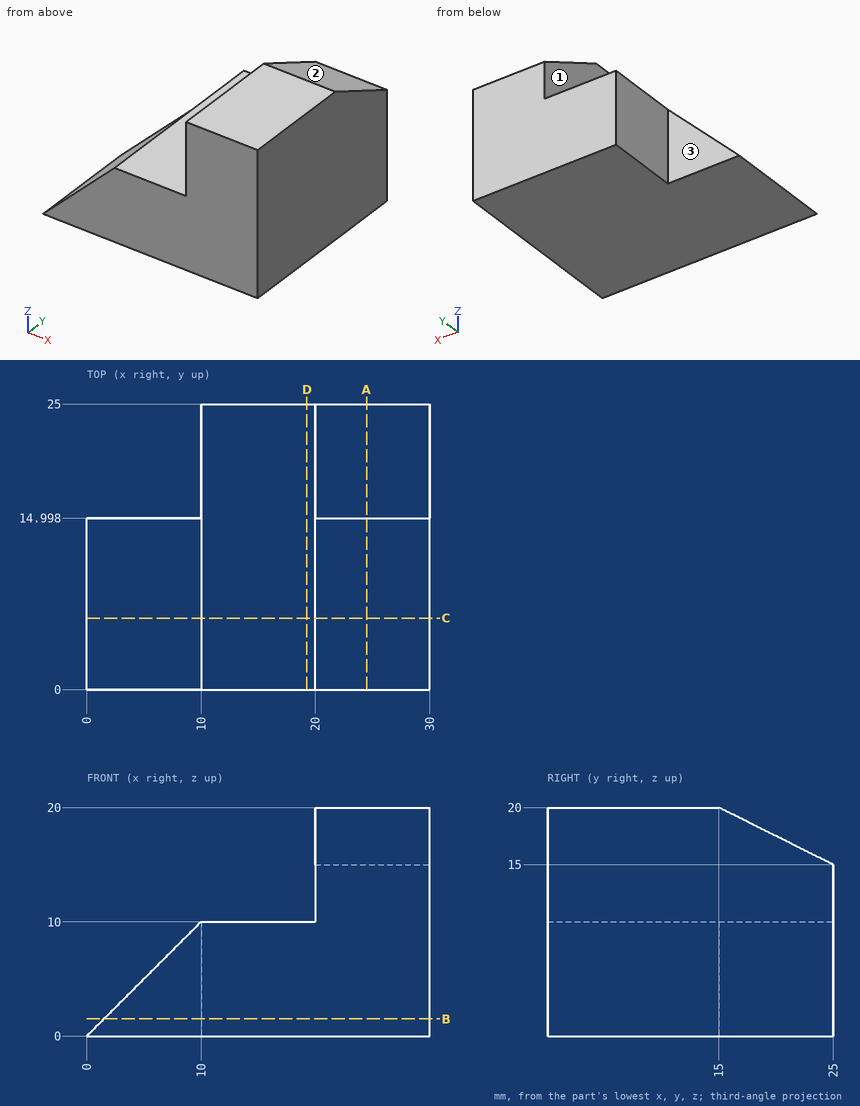
Input: dimensioned drawing with shaded views. Units: mm. Origin: part minimum x, y, z. A direction names the side the tool comes from. Coordinates: 2 decimals unless noted, no trailing zeros. Loops run counter-clockwise (first coordinate to the right, second up) from the corner with the lowest first, then second, coordinate; pieces in that order, holes last. Notation, with made-up numbers: M -23,-10 L 11,-10 A28 cw 11,15 Z; hole C 28,89 d7. An arc over 180 degrees is marked long. One line per item, written item: value. Start each with the question number.
1) Cut plane C-C (y = 6.25). Return loops of the section in (x, z).
2) Reachability of the marked faces 1, 2 and 3 from +Z, -Z, +X, -X, +Y, -Y: full face, straight path, thin tool, end or side. Return the list, or none.
3) Material intervals for L1, parallel to Z at x = 14.25, y = 17.25; L2, parallel to X at y = 21, z = 15.5; L3, parallel to X at y = 15.5, z = 2.25, sorted ascending. Write a range as from..to.
4) Cut plane D-D (x = 19.25). Return loops of the section in (y, z).
5) Cut plane B-B (z = 1.5). Return loops of the section in (x, y).
6) Pin query (flat end, axial travel): P1, Ø3, axis at y = 12.5, z = 3.5, coming from the -X side; P2, Ø3, axis at x = 7, z = 7, coming from the +Y side; P3, Ø8, axis at x = 14, y = 12, coming from the +Z side. Return the tip coordinate at first contact, or that it passes through.
7) Cut plane A-A (x = 24.5). Return loops of the section in (y, z).
Evaluation:
1. outline: M 0,0 L 30,0 L 30,20 L 20,20 L 20,10 L 10,10 Z
2. face 1: +Z, -X, +Y, -Y
2. face 2: +Z, +X, -X, +Y
2. face 3: +Z, -Z, -X, +Y
3. L1: 0..10
3. L2: 20..30
3. L3: 10..30
4. outline: M 0,0 L 25,0 L 25,10 L 0,10 Z
5. outline: M 1.5,0 L 30,0 L 30,25 L 10,25 L 10,15 L 1.5,15 Z
6. P1: x = 2
6. P2: y = 15
6. P3: z = 10
7. outline: M 0,0 L 25,0 L 25,15 L 15,20 L 0,20 Z
